from build123d import *

# Parameters (mm, degrees)
F1_DEPTH = 101.6


with BuildPart() as f1:
    # F0 (on Right) → F1 (new body)
    with BuildSketch(Plane.YZ):
        Polygon((561.29576, 313.291845), (-48.30424, 313.291845), (-48.30424, 211.691845), (536.716133, 211.691845), (2068.830831, -575.708155), (2291.102677, -575.708155), (2085.29576, -469.937767), (2021.611301, -437.208401), (1987.724537, -419.79297), (1780.49576, -313.291845), (1716.811301, -280.562478), (1475.69576, -156.645922), (1412.011301, -123.916556), (1170.89576, 0), (1107.211301, 32.729366), (866.09576, 156.645922), (802.411301, 189.375289), (772.271858, 204.864858), align=None)
    extrude(amount=F1_DEPTH)


solid = f1.part
Check sheet for the modelled part. Datum: model origin and axes. Units: mm. A direction names the side the tool comes from. Round coordinates to 2 decimals unless told otherwise and drop trailing zeros. Order: outer loops, then holes, each group sorted by start corner. A loop starts at its lowest first (then second) coordinate and runs counter-clockwise, first axis right, second up.
(1) Go/stop test with flat-tipped pins: P1, Ø1.5, axis at x = 25, z = -360, coming from the -Y side; P2, Ø8, axis at x = 38.5, z = 6, coming from the -Y side; P3, Ø5, axis at x = 39, y = 1018, coming from the +Z side. Record where each tip stops, or that it passes through.
(2) Cross-section at A-A, the plane x = 30. Enter the section's corners in (y, z), and give its area (3 significant figures).
(3) Scan lines: probe 1 along Z at (x, y) = (28.5, 54.5); probe 2 along Y at (x, z) = (7.5, -425); probe 3 along Y at (x, z) = (22, -170). Record each from-to range of solid material in increasing order.
(4) Access from +Z, -Z, +X, -X, +Y, -Y to the whole of each face (thin tool, end or side, straight path). Record for faces 1 (the flat face through (50, 2178, -575.708)), 2 (the flat face through (50, 240, 211.692)).
(5) Cross-section at B-B, the plane y = 332. Enter the section's corners in (x, z), and give its area (3 significant figures).
(6) Cross-section at C-C, the plane z = -181. Enter the section's corners in (x, y), and give its area (3 significant figures).
Check sheet entries:
1. P1: stops at y = 1647.65
1. P2: stops at y = 929.17
1. P3: stops at z = 79.86
2. outline: (-48.3, 211.69) - (536.72, 211.69) - (2068.83, -575.71) - (2291.1, -575.71) - (561.3, 313.29) - (-48.3, 313.29) - close
2. area: 247,000 mm2
3. probe 1: z = 211.69 to 313.29
3. probe 2: y = 1775.58 to 1997.86
3. probe 3: y = 1279.41 to 1501.68
4. face 1: -Z, +X, -X, +Y, -Y
4. face 2: -Z, +X, -X, -Y
5. outline: (0, 211.69) - (101.6, 211.69) - (101.6, 313.29) - (0, 313.29) - close
5. area: 10,300 mm2
6. outline: (0, 1300.81) - (101.6, 1300.81) - (101.6, 1523.08) - (0, 1523.08) - close
6. area: 22,600 mm2
